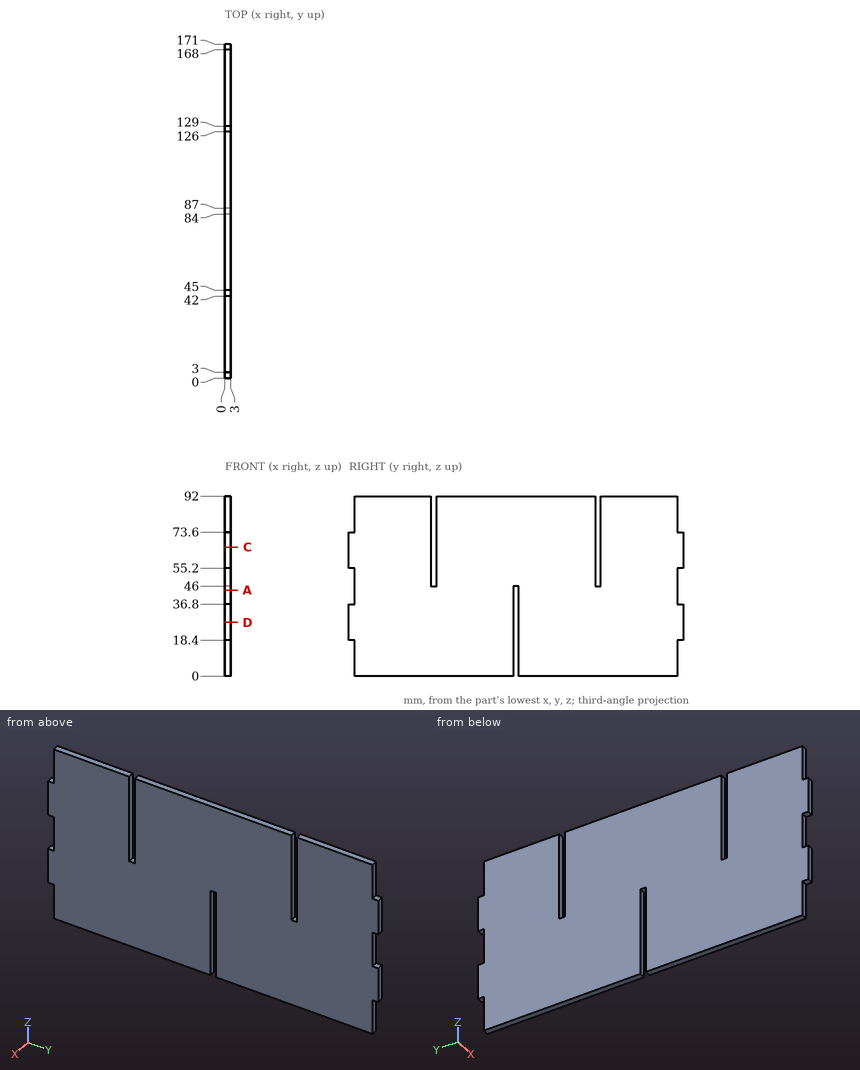
Input: dimensioned drawing with shaded views. Units: mm. Origin: part minimum x, y, z. Round coordinates to 2 decimals unless told otherwise and drop trailing zeros. Loops run counter-clockwise (first coordinate to the right, second up) from the corner with the lowest first, then second, coordinate; pieces in that order, holes last. Notation, with made-up numbers: (63, 46.25) -> (100, 46.25) arc R20 cw to (100, 83.25) -> close; hole circle Ø9 at (16.5, -2.75). An arc over 180 degrees is marked (long way). Use one line per item in the form item = value. Start each with the question number.
1) Section D-D on z = 27.5. Output: boundary loops of the cut face in (x, y).
2) Section C-C on z = 66. Output: boundary loops of the cut face in (x, y).
3) Section A-A on z = 44. Output: boundary loops of the cut face in (x, y), then the cut area to 3 significant figures.
4) First-contact query: P1, Ø8, axis at y = 44.5, z = 80.5, coming from the -X side; P2, Ø1.5, axis at x = 1, z = 80, coming from the -Y side; P3, Ø0.9, axis at x = 2, z = 79, coming from the +Y side; P4, Ø1.5, axis at x = 1.5, y = 169, coming from the +Z side. Flat tips, straight axial feed; report the tip coordinate or a pass-through.
5) Line query: L1, parallel to Y at x = 0.4, z = 66; L2, parallel to Y at x = 1.5, z = 75; L3, parallel to Y at x = 0.25, z = 23.5. Output: solid intervals per line, ascending.
Response:
q1.outline = (0, 0) -> (3, 0) -> (3, 84) -> (0, 84) -> close; (0, 87) -> (3, 87) -> (3, 171) -> (0, 171) -> close
q2.outline = (0, 0) -> (3, 0) -> (3, 42) -> (0, 42) -> close; (0, 45) -> (3, 45) -> (3, 126) -> (0, 126) -> close; (0, 129) -> (3, 129) -> (3, 171) -> (0, 171) -> close
q3.outline = (0, 3) -> (3, 3) -> (3, 84) -> (0, 84) -> close; (0, 87) -> (3, 87) -> (3, 168) -> (0, 168) -> close
q3.area = 486 mm^2
q4.P1 = 0
q4.P2 = 3
q4.P3 = 168
q4.P4 = 73.6
q5.L1 = 0 to 42, 45 to 126, 129 to 171
q5.L2 = 3 to 42, 45 to 126, 129 to 168
q5.L3 = 0 to 84, 87 to 171
